Autodesk Inventor part; units mm, degrees
ref_plane "Plano de trabajo1" through (-250, 0, 500) normal (1, 0, 0) x (0, 0, -1)
ref_plane "YZ Plane" through (0, 0, 0) normal (1, 0, 0) x (0, 1, 0)
ref_plane "XZ Plane" through (0, 0, 0) normal (0, 1, 0) x (-1, 0, 0)
sketch "Boceto1" plane through (0, 0, 0) normal (0, 1, 0) x (-1, 0, 0)
  line L0 (0, 0) -> (0, -500) construction
  line L1 (0, -500) -> (500, -500) construction
  line L2 (500, -500) -> (500, 500) construction
  line L3 (500, 500) -> (0, 500) construction
  line L4 (0, 500) -> (0, 0) construction
  line L5 (500, 500) -> (0, 500)
  line L6 (0, 500) -> (0, -500)
  line L7 (0, -500) -> (500, -500)
  line L8 (500, -500) -> (500, 500)
  dimension "d0" = 500
  dimension "d1" = 500
  dimension "d2" = 1000
extrude "Extrusión1" add sketch "Boceto1" along normal blind 20
sketch "Boceto2" plane through (0, 20, 0) normal (0, 1, 0) x (1, 0, 0)
  line L0 (0, 500) -> (-500, 500) construction
  line L1 (-250, 500) -> (-250, -500) construction
  line L2 (-500, -500) -> (0, -500) construction
  line L3 (-265.9292, 440.1456) -> (-234.905, 440.1456)
  line L4 (-234.905, 440.1456) -> (-234.905, 415.7448)
  line L5 (-234.905, 415.7448) -> (-265.9292, 415.7448)
  line L6 (-265.9292, 415.7448) -> (-265.9292, 440.1456)
  point P0 (0, 0)
extrude "Extrusión2" add sketch "Boceto2" along normal blind 1000
mirror "Simetría1" about plane through (0, 0, 0) normal (0, 0, 1) of "Extrusión2"
sketch "Boceto4" plane through (-265.9292, 20, 440.1456) normal (0, 0, 1) x (1, 0, 0)
  line L0 (31.0242, 0) -> (31.0242, 1000) construction
  line L1 (31.0242, 379.2693) -> (193.3148, 0) construction
  line L2 (31.0242, 314.0177) -> (165.3935, 0) construction
  line L3 (-234.0708, 0) -> (265.9292, 0) construction
  line L4 (31.0242, 379.2693) -> (193.3148, 0)
  line L5 (165.3935, 0) -> (31.0242, 314.0177)
  line L6 (31.0242, 379.2693) -> (31.0242, 314.0177)
  line L7 (165.3935, 0) -> (193.3148, 0)
  point P0 (265.9292, -20)
extrude "Extrusión3" add sketch "Boceto4" against normal up to surface (24.4008 mm away)
ref_plane "Plano de trabajo1" through (-250, 0, 500) normal (1, 0, 0) x (0, 0, -1)
mirror "Simetría2" about plane through (-250, 0, 500) normal (1, 0, 0) of "Extrusión3"
mirror "Simetría3" about plane through (0, 0, 0) normal (0, 0, 1) of "Extrusión3", "Simetría2"
sketch "Boceto5" plane through (0, 20, 0) normal (0, 1, 0) x (1, 0, 0)
  line L0 (-72.6144, 415.7448) -> (-234.905, 415.7448) construction
  line L1 (-78.0914, 415.7448) -> (-78.0914, 405.899) construction
  line L2 (-95.8718, 415.7448) -> (-95.8718, 405.899) construction
  line L3 (-78.0914, 415.7448) -> (-95.8718, 415.7448)
  line L4 (-95.8718, 0) -> (-95.8718, 415.7448)
  line L5 (-78.0914, 415.7448) -> (-78.0914, 0)
  line L6 (-78.0914, 0) -> (-78.0914, -415.7448)
  line L7 (-100.5357, -415.7448) -> (-72.6144, -415.7448)
  line L8 (-95.8718, 0) -> (-95.8718, -415.7448)
  line L9 (-78.0914, -415.7448) -> (-95.8718, -415.7448)
  point P0 (0, 0)
extrude "Extrusión4" cut sketch "Boceto5" against normal blind 5
mirror "Simetría4" about plane through (-250, 0, 500) normal (1, 0, 0) of "Extrusión4"
sketch "Boceto6" plane through (0, 20, 0) normal (0, 1, 0) x (1, 0, 0)
  line L0 (-265.9292, 415.7448) -> (-234.905, 415.7448) construction
  line L1 (-239.0903, 415.7448) -> (-239.0903, 391.5107) construction
  line L2 (-260.3339, 415.7448) -> (-260.3339, 390.2687) construction
  line L3 (-265.9292, -415.7448) -> (-234.905, -415.7448) construction
  line L4 (-239.0903, 415.7448) -> (-260.3339, 415.7448) construction
  line L5 (-260.3339, -415.7448) -> (-239.0903, -415.7448) construction
  line L6 (-239.0903, -415.7448) -> (-260.3339, -415.7448)
  line L7 (-239.0903, 415.7448) -> (-260.3339, 415.7448)
  line L8 (-239.0903, 65.2159) -> (-260.3339, 65.2159)
  line L9 (-239.0903, -72.6288) -> (-260.3339, -72.6288)
  line L10 (-239.0903, -415.7448) -> (-239.0903, -72.6288)
  line L11 (-239.0903, 65.2159) -> (-239.0903, 415.7448)
  line L12 (-260.3339, 415.7448) -> (-260.3339, 65.2159)
  line L13 (-260.3339, -72.6288) -> (-260.3339, -415.7448)
  point P0 (0, 0)
extrude "Extrusión5" cut sketch "Boceto6" against normal blind 5
sketch "Boceto7" plane through (0, 20, 0) normal (0, 1, 0) x (1, 0, 0)
  line L0 (-224.1946, 33.7447) -> (-276.8566, 33.7447)
  line L1 (-276.8566, 33.7447) -> (-276.8566, -31.5828)
  line L2 (-276.8566, -31.5828) -> (-224.1946, -31.5828)
  line L3 (-224.1946, -31.5828) -> (-224.1946, 33.7447)
  point P0 (0, 0)
extrude "Extrusión6" cut sketch "Boceto7" against normal blind 10
sketch "Boceto8" plane through (0, 10, 0) normal (0, 1, 0) x (1, 0, 0)
  point P0 (0, 0)
  point P1 (-230.6615, -24.5924)
hole "Agujero1" at (-230.6615, 10, 24.5924) direction (0, -1, 0) diameter 3 end through all
mirror "Simetría5" about plane through (-250, 0, 500) normal (1, 0, 0) of "Agujero1"
mirror "Simetría6" about plane through (0, 0, 0) normal (0, 0, 1) of "Agujero1", "Simetría5"
sketch "Boceto9" plane through (-265.9292, 397.3198, -415.7448) normal (0, 0, 1) x (1, 0, 0)
  line L0 (0, 0) -> (0, 622.6802)
  line L1 (31.0242, 1.9495) -> (31.0242, 622.6802)
  arc A0 (0, 595.7054) -> (31.0242, 595.8449) centre (15.4643, 606.4176) ccw
  line L2 (0, 595.7054) -> (0, 599.8174)
  line L3 (31.0242, 595.8449) -> (31.0242, 599.8174)
  arc A1 (0, 599.8174) -> (31.0242, 599.8174) centre (15.5121, 611.2009) ccw
  point P0 (265.9292, -397.3198)
extrude "Extrusión7" add sketch "Boceto9" along normal blind 40
mirror "Simetría7" about plane through (0, 0, 0) normal (0, 0, 1) of "Extrusión7"
properties part number "Structure_provisional"
CAD build for the part. Positions are in the model's coordinates, mm. A direction names the side the tool comes from. Give positions to 0.01 mm unless a question says otherwise; leave off trailing zeros. Order: outer loops, then holes, each group sorted by start corner. A loop starts at its lowest first (then second) coordinate and runs counter-clockwise, first axis right, second up. Notation, with made-up numbers: (74.5, -34.75) - (130.5, -34.75) arc R16 cw to (130.5, -30.75) - close; hole circle Ø7 at (87.25, -28). An arc over 180 degrees is marked (long way). Write each question's results on one line, items separated by ' | '.
1. Probe L1, parallel to Z at x = -170, y = 216.5; L2, parallel to Y at x = -21.5, z = 82.5; L3, parallel to Y at x = -81, z = -87. List the from-to ranges inside material, lowest first. Write a range as from..to.
Calculated:
L1: z = -440.15..-415.74, 415.74..440.15 | L2: y = 0..20 | L3: y = 0..15
2. Saw through at A-A on z = -84. List the corners of the cut face in (x, y).
Calculated:
outline: (-500, 0) - (0, 0) - (0, 20) - (-78.09, 20) - (-78.09, 15) - (-95.87, 15) - (-95.87, 20) - (-239.09, 20) - (-239.09, 15) - (-260.33, 15) - (-260.33, 20) - (-404.13, 20) - (-404.13, 15) - (-421.91, 15) - (-421.91, 20) - (-500, 20) - close
3. Saw through at B-B on y = 834. List the corners of the cut face in (x, z) (3 decimals).
Calculated:
outline: (-265.929, -440.146) - (-234.905, -440.146) - (-234.905, -415.745) - (-265.929, -415.745) - close; (-265.929, 415.745) - (-234.905, 415.745) - (-234.905, 440.146) - (-265.929, 440.146) - close
4. Saw through at C-C on x = -151. List the corners of the cut face in (y, z).
Calculated:
outline: (0, -500) - (20, -500) - (20, 500) - (0, 500) - close; (137.93, -440.15) - (203.19, -440.15) - (203.19, -415.74) - (137.93, -415.74) - close; (137.93, 415.74) - (203.19, 415.74) - (203.19, 440.15) - (137.93, 440.15) - close
5. Pull direction Z, two halves, no side cores. Call faces 5 (the face through (-234.905, 175, -428)), 6 (the face through (-249, 411, -440.146)), 7 (the face through (-250.16, 989.28, -396.02)): released by +Z, released by -Z, zero draft, split by the parting line, or undercut.
Calculated:
face 5: zero draft | face 6: released by -Z | face 7: undercut
6. Saw through at D-D on y = 116.5. List the corners of the cut face in (x, z) (3 decimals).
Calculated:
outline: (-386.093, -440.146) - (-358.172, -440.146) - (-358.172, -415.745) - (-386.093, -415.745) - close; (-386.093, 415.745) - (-358.172, 415.745) - (-358.172, 440.146) - (-386.093, 440.146) - close; (-265.929, -440.146) - (-234.905, -440.146) - (-234.905, -415.745) - (-265.929, -415.745) - close; (-265.929, 415.745) - (-234.905, 415.745) - (-234.905, 440.146) - (-265.929, 440.146) - close; (-141.828, -440.146) - (-113.907, -440.146) - (-113.907, -415.745) - (-141.828, -415.745) - close; (-141.828, 415.745) - (-113.907, 415.745) - (-113.907, 440.146) - (-141.828, 440.146) - close
7. Pin check, flat tips, straight feed: pin 1 (1.5 mm diameter, centred on x = -184.5, z = -164.5, fed in from +Y); pin 2 (1.5 mm diameter, centred on y = 18.5, z = -59, fed in from +X); pin 3 (7.5 mm diameter, centred on y = 222, z = 426.5, fed in from +X); pin 4 (14 mm diameter, centred on x = -413, z = 65.5, fed in from +Y). Stop position of each tip, or through.
Calculated:
pin 1: stops at y = 20 | pin 2: stops at x = 0 | pin 3: stops at x = -157.45 | pin 4: stops at y = 15
8. 3-axis set-ups, long thin cutter, end or side, ignore diameter. For faces 1 (the face through (-250.636, 984.926, 396.025)), 2 (the face through (-250.67, 989.28, 396.02)), 3 (the face through (-265.929, 707, 427)), 4 (the face through (-333.63, 173.85, -428.12)): which of +Z, -Z, +X, -X, +Y, -Y reach the whole face in a straight line?
Calculated:
face 1: none | face 2: +Y | face 3: +Z, -Z, -X, +Y | face 4: +Z, -Z
